Print and shaded views of the part. All mm, measured from the part's lowest x, y and z. A direction names the side the tool comes from. Give positions to 0.01 mm unless a question says otherwise; leave off trailing zeros. Order: outer loops, then holes, each group sorted by start corner. A loop starts at its lowest first (then second) coordinate and runs counter-clockwise, first axis right, second up. Notation, with made-up numbers: (54.5, 82) -> (88.5, 82) arc R22 ccw to (88.5, 100) -> close; hole circle Ø2 at (3.5, 66.25). An arc over 180 degrees is marked (long way). One line per question, with ' | ' between items. Start each with the question number.
(1) Drill centre lines: L1, parallel to Z at x = 20, y = 5.25 (1 decimal); L2, parallel to Y at x = 32, z = 37.5 (3 decimals); L3, parallel to X at y = 3.25, z = 26. Where is each one in solid material? Low to high. Write a range as from..to.
(2) Which spindle directions (+Z, -Z, +X, -X, +Y, -Y) get a long thin tool onto all of the face, cutting with end or side? Do the marked faces 4 and 5. Say none if no direction does.
(3) Cut at B-B (x = 20). Give the cut face in (y, z) (1 decimal), then the cut area to 3 significant figures.
(4) Cut at D-D (x = 10). Give the cut face in (y, z) (3 decimals), then the cut area to 3 significant figures.
(5) Pin check, flat tips, straight feed: pin 1 Ø3 at (x, z) = (36, 26.5) entering from -Y (3 decimals); pin 2 Ø6 at (x, y) = (23.5, 3) entering from -Z; pin 3 Ø1.5 at (x, y) = (24.5, 4.5) entering from +Z. Stop position of each tip, or through.
(6) Cut at A-A (z = 20). Give the cut face in (x, y) (1 decimal).
(7) Pull direction Z, two halves, no side cores. Call the marked faces 1, 2 and 3: +Z half, -Z half, draft (parallel to the pull), parting line (faces both ways), or undercut.
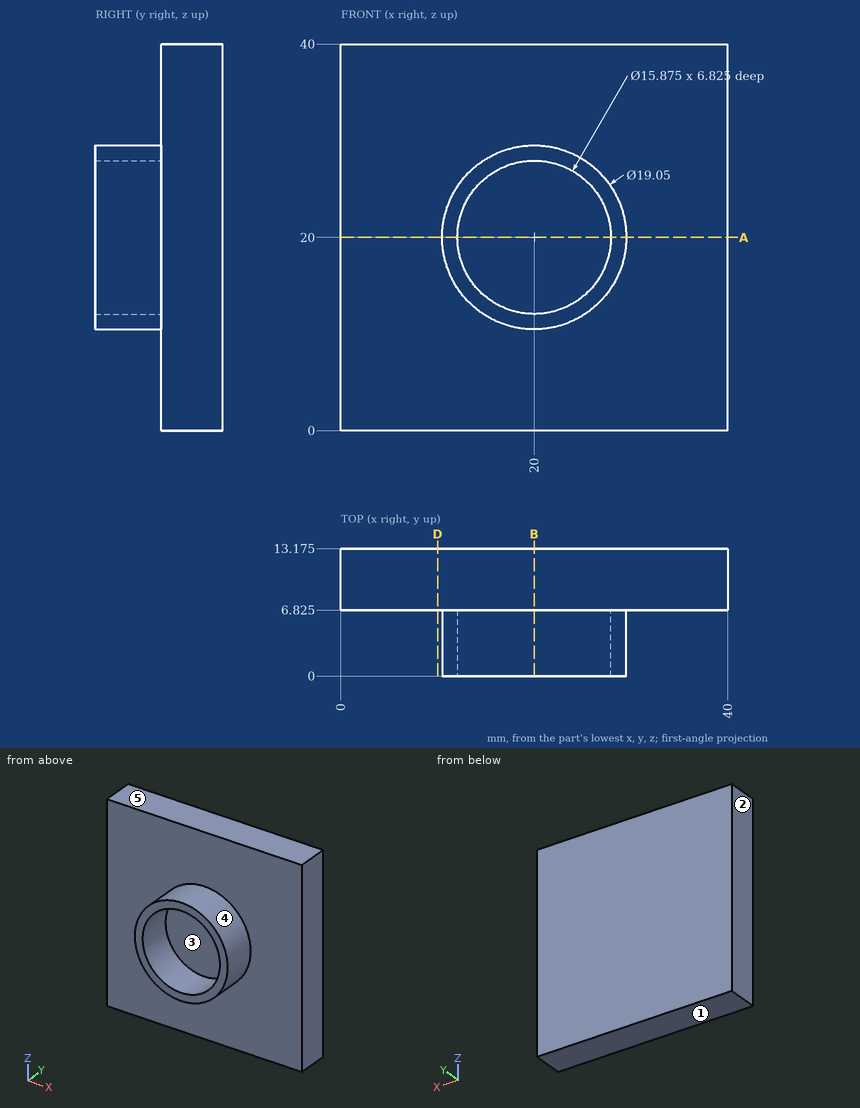
Result set:
1) L1: z = 10.5..12.1, 27.9..29.5 | L2: y = 6.825..13.175 | L3: x = 12.6..14.8, 25.2..27.4
2) face 4: -Y | face 5: +Z, +X, -X, +Y, -Y
3) outline: (0, 10.5) -> (6.8, 10.5) -> (6.8, 0) -> (13.2, 0) -> (13.2, 40) -> (6.8, 40) -> (6.8, 29.5) -> (0, 29.5) -> (0, 27.9) -> (6.8, 27.9) -> (6.8, 12.1) -> (0, 12.1) -> close | area: 276 mm2
4) outline: (6.825, 0) -> (13.175, 0) -> (13.175, 40) -> (6.825, 40) -> close | area: 254 mm2
5) pin 1: stops at y = 6.825 | pin 2: stops at z = 10.49 | pin 3: stops at z = 28.76
6) outline: (0, 6.8) -> (10.5, 6.8) -> (10.5, 0) -> (12.1, 0) -> (12.1, 6.8) -> (27.9, 6.8) -> (27.9, 0) -> (29.5, 0) -> (29.5, 6.8) -> (40, 6.8) -> (40, 13.2) -> (0, 13.2) -> close
7) face 1: -Z half | face 2: draft | face 3: undercut
